Autodesk Inventor part; units mm, degrees
ref_plane "YZ Plane" through (0, 0, 0) normal (1, 0, 0) x (0, 1, 0)
ref_plane "XZ Plane" through (0, 0, 0) normal (0, 1, 0) x (-1, 0, 0)
ref_plane "XY Plane" through (0, 0, 0) normal (0, 0, 1) x (1, 0, 0)
sketch "Sketch1" plane through (0, 0, 0) normal (0, 0, 1) x (1, 0, 0)
  line L0 (0, 0) -> (25.4, 0)
  line L1 (25.4, 0) -> (25.4, 50.8)
  line L2 (25.4, 50.8) -> (0, 50.8)
  line L3 (0, 50.8) -> (0, 0)
  line L4 (1.5875, 49.2125) -> (23.8125, 49.2125)
  line L5 (23.8125, 49.2125) -> (23.8125, 1.5875)
  line L6 (23.8125, 1.5875) -> (1.5875, 1.5875)
  line L7 (1.5875, 1.5875) -> (1.5875, 49.2125)
  dimension "d0" = 25.4
  dimension "d1" = 50.8
  dimension "d2" = 1.5875
extrude "Extrusion1" add sketch "Sketch1" along normal blind 685.8
sketch "Sketch2" plane through (25.4, 0, 0) normal (1, 0, 0) x (0, 0, -1)
  line L0 (0, 49.2125) -> (0, 1.5875) construction
  line L1 (0, 25.4) -> (-95.25, 25.4) construction
  line L2 (0, 25.4) -> (-209.55, 25.4) construction
  line L3 (0, 25.4) -> (-288.925, 25.4) construction
  circle A0 centre (-95.25, 25.4) radius 19.05
  circle A1 centre (-209.55, 25.4) radius 19.05
  circle A2 centre (-288.925, 25.4) radius 19.05
  line L4 (0, 50.8) -> (-685.8, 50.8) construction
  line L5 (-342.9, 50.8) -> (-342.9, -48.6328) construction
  circle A3 centre (-590.55, 25.4) radius 19.05
  circle A4 centre (-476.25, 25.4) radius 19.05
  circle A5 centre (-396.875, 25.4) radius 19.05
  point P0 (0, 0)
  dimension "d5" = 95.25
  dimension "d6" = 209.55
  dimension "d7" = 288.925
  dimension "d8" = 38.1
  dimension "d9" = 38.1
  dimension "d10" = 38.1
extrude "Extrusion2" cut sketch "Sketch2" against normal blind 685.8
sketch "Sketch3" plane through (0, 50.8, 0) normal (0, 1, 0) x (1, 0, 0)
  line L0 (23.8125, 0) -> (1.5875, 0) construction
  line L1 (12.7, 0) -> (12.7, -38.1) construction
  line L2 (12.7, -38.1) -> (12.7, -63.5) construction
  line L3 (12.7, -63.5) -> (12.7, -139.7) construction
  line L4 (25.4, -685.8) -> (0, -685.8) construction
  line L5 (12.7, -685.8) -> (12.7, -647.7) construction
  line L6 (12.7, -647.7) -> (12.7, -622.3) construction
  line L7 (12.7, -622.3) -> (12.7, -546.1) construction
  circle A0 centre (12.7, -647.7) radius 2.5797
  circle A1 centre (12.7, -622.3) radius 2.5797
  circle A2 centre (12.7, -546.1) radius 2.5797
  circle A3 centre (12.7, -139.7) radius 2.5797
  circle A4 centre (12.7, -63.5) radius 2.5797
  circle A5 centre (12.7, -38.1) radius 2.5797
  line L8 (12.7, -685.8) -> (12.7, -673.1) construction
  line L9 (12.7, 0) -> (12.7, -12.7) construction
  circle A6 centre (12.7, -12.7) radius 2.5797
  circle A7 centre (12.7, -673.1) radius 2.5797
  point P0 (0, 0)
  dimension "d13" = 38.1
  dimension "d14" = 25.4
  dimension "d15" = 76.2
  dimension "d16" = 38.1
  dimension "d17" = 25.4
  dimension "d18" = 76.2
  dimension "d19" = 5.1594
  dimension "d24" = 12.7
  dimension "d25" = 12.7
extrude "Extrusion5" cut sketch "Sketch3" against normal blind 215.9
sketch "Sketch4" plane through (25.4, 0, 0) normal (1, 0, 0) x (0, 0, -1)
  line L0 (-685.8, 0) -> (-422.3766, 0) construction
  line L1 (0, 0) -> (-685.8, 0) construction
  line L2 (-422.3766, 0) -> (-422.3766, 12.8524) construction
  line L3 (-422.3766, 12.8524) -> (-422.3766, 38.2524) construction
  line L4 (-422.3766, 38.2524) -> (-371.5766, 38.2524) construction
  line L5 (-371.5766, 38.2524) -> (-371.5766, 12.8524) construction
  line L6 (0, 50.8) -> (-685.8, 50.8) construction
  line L7 (-342.9, 50.8) -> (-342.9, 0) construction
  circle A0 centre (-422.3766, 38.2524) radius 2.5781
  circle A1 centre (-422.3766, 12.8524) radius 2.5781
  circle A2 centre (-371.5766, 12.8524) radius 2.5781
  circle A3 centre (-371.5766, 38.2524) radius 2.5781
  circle A4 centre (-263.4234, 38.2524) radius 2.5781
  circle A5 centre (-263.4234, 12.8524) radius 2.5781
  circle A6 centre (-314.2234, 12.8524) radius 2.5781
  circle A7 centre (-314.2234, 38.2524) radius 2.5781
  dimension "d16" = 38.1
  dimension "d17" = 25.4
  dimension "d18" = 76.2
  dimension "d19" = 5.1594
  dimension "d24" = 12.7
  dimension "d28" = 263.4234
  dimension "d29" = 12.8524
  dimension "d30" = 25.4
  dimension "d31" = 50.8
  dimension "d32" = 25.4
  dimension "d33" = 5.1562
extrude "Extrusion6" cut sketch "Sketch4" against normal blind 215.9
properties part number "driveline 1x2"
Here's how the part is built. I have some questions about the finished solid (model axes, mm). A direction names the side the tool comes from. Round coordinates to 2 decimals unless told otherwise and drop trailing zeros. Order: outer loops, then holes, each group sorted by start corner. A loop starts at its lowest first (then second) coordinate and runs counter-clockwise, first axis right, second up. Notation, with made-up numbers: (76, -37.75) -> (124, -37.75) arc R29 cw to (124, -3.75) -> close; hole circle Ø6 at (-39, 8). An arc over 180 degrees is marked (long way). Use a Markdown table: item, result. Add a question column.
(1) For pin 1 Ø3 at (y, z) = (12.85, 371.58) entering from +X, with a flat end and sliding along its axis, tell me the tip position at first contact or that it passes through.
(2) Suppose I cut it at C-C, the plane z = 94. Please give me the cut outline in (x, y).
(3) I need wall thicknesses on line 1 along X through (y, z) = (0.65, 647.7); line 2 along Y through (x, z) = (10, 356.5); line 3 along X through (y, z) = (24, 319). Which ranges of each line are inside material? Lowest first, please.
(4) Suppose I cut it at A-A, the plane z = 476.25. Please give me the cut outline in (x, y).
(5) Suppose I cut it at B-B, the plane y = 25.4. Count the separate pieces of the cut face and the enclosed holes in it, and give its area (3 significant figures).
(6) For faces 4 (the face through (13, 0, 338)), 5 (the face through (13, 49.212, 338)), which set-ups out of +Z, -Z, +X, -X, +Y, -Y let a thin tool reach every point of the face, with its end or its side?
(7) If we mould it in two halves opening along Y, with no side actions, what happens to faces 1 (the face through (13, 50.8, 338)), 2 (the face through (13, 1.588, 338)), 3 (the face through (25.4, 25, 338))? For each: released by +Y, released by -Y, zero draft, split by the parting line, or undercut.
Verdict:
| question | item | result |
|---|---|---|
| 1 | pin 1 | through |
| 2 | outline | (0, 0) -> (25.4, 0) -> (25.4, 6.39) -> (23.81, 6.39) -> (23.81, 1.59) -> (1.59, 1.59) -> (1.59, 6.39) -> (0, 6.39) -> close; (0, 44.41) -> (1.59, 44.41) -> (1.59, 49.21) -> (23.81, 49.21) -> (23.81, 44.41) -> (25.4, 44.41) -> (25.4, 50.8) -> (0, 50.8) -> close |
| 3 | line 1 | 0 to 10.12, 15.28 to 25.4 |
| 3 | line 2 | 0 to 1.59, 49.21 to 50.8 |
| 3 | line 3 | 0 to 1.59, 23.81 to 25.4 |
| 4 | outline | (0, 0) -> (25.4, 0) -> (25.4, 6.35) -> (23.81, 6.35) -> (23.81, 1.59) -> (1.59, 1.59) -> (1.59, 6.35) -> (0, 6.35) -> close; (0, 44.45) -> (1.59, 44.45) -> (1.59, 49.21) -> (23.81, 49.21) -> (23.81, 44.45) -> (25.4, 44.45) -> (25.4, 50.8) -> (0, 50.8) -> close |
| 5 | separate pieces | 14 |
| 5 | enclosed holes | 0 |
| 5 | area | 1,450 mm2 |
| 6 | face 4 | +Z, -Z, +X, -X, -Y |
| 6 | face 5 | +Z, -Z |
| 7 | face 1 | released by +Y |
| 7 | face 2 | undercut |
| 7 | face 3 | zero draft |
